Source: CAD feature listing. Evaluate the final solid. Frame: model axes, mm. A direction names the side the tool comes from. Give positions to 0.01 mm unless a question says otherwise; leave off trailing zeros. Loops run counter-clockwise (first coordinate to the right, second up) from the corner with the lowest first, then second, coordinate; pieces in that order, holes last.
from build123d import *

# Parameters (mm, degrees)
BOSS_EXTRUDE1_DEPTH = 50
SKETCH2_W           = 9
SKETCH2_H           = 2
BOSS_EXTRUDE2_DEPTH = 10
SKETCH3_R           = 3.15
CUT_EXTRUDE1_DEPTH  = 1
BOSS_EXTRUDE3_DEPTH = 50
SKETCH5_W           = 5
SKETCH5_H           = 2
BOSS_EXTRUDE4_DEPTH = 1
SKETCH6_R           = 4.5
SKETCH6_R_2         = 2.5
CUT_EXTRUDE2_DEPTH  = 1
CUT_EXTRUDE3_DEPTH  = 65.610577824


with BuildPart() as part:
    # Sketch1 → Boss-Extrude1 (new body)
    with BuildSketch(Plane(origin=(0, 0, 0), x_dir=(1, 0, 0), z_dir=(0, 1, 0))):
        Polygon((0, 0), (0, -6), (7, -6), (7, -4), (2, -4), (2, -2), (9, -2), (9, 0), align=None)
    extrude(amount=BOSS_EXTRUDE1_DEPTH)

    # Sketch2 → Boss-Extrude2 (add)
    with BuildSketch(Plane(origin=(0, 50, 0), x_dir=(1, 0, 0), z_dir=(0, 1, 0))):
        with Locations((4.5, -1)):
            Rectangle(SKETCH2_W, SKETCH2_H)
    extrude(amount=BOSS_EXTRUDE2_DEPTH)

    # Sketch3 → Cut-Extrude1 (cut)
    with BuildSketch(Plane(origin=(0, 0, 0), x_dir=(-1, 0, 0), z_dir=(0, 0, -1))):
        with Locations((-5.5, 55)):
            Circle(SKETCH3_R)
    extrude(amount=-CUT_EXTRUDE1_DEPTH, mode=Mode.SUBTRACT)

    # Sketch4 → Boss-Extrude3 (add)
    with BuildSketch(Plane.XZ):
        Polygon((17.441727636, 16.441727636), (7, 6), (0, 13), (10.857923623, 23.349178451), align=None)
        Polygon((7, 6), (0, 13), (0, 6), align=None)
    extrude(amount=-BOSS_EXTRUDE3_DEPTH)

    # Sketch5 → Boss-Extrude4 (add)
    with BuildSketch(Plane.XZ):
        with Locations((4.5, 3)):
            Rectangle(SKETCH5_W, SKETCH5_H)
    extrude(amount=-BOSS_EXTRUDE4_DEPTH)

    # Sketch6 → Cut-Extrude2 (cut)
    # profile 1 of 2: a face of its own
    with BuildSketch(Plane(origin=(17.350446553, 0, 16.537495917), x_dir=(0.6899452300561162, 0, -0.7238615748351429), z_dir=(0.7238615748351429, 0, 0.6899452300561162))):
        with Locations((-4.638949273, 40)):
            Circle(SKETCH6_R)
        with Locations((-4.638949273, 40)):
            Circle(SKETCH6_R_2, mode=Mode.SUBTRACT)
    # profile 2 of 2: a face of its own
    with BuildSketch(Plane(origin=(17.350446553, 0, 16.537495917), x_dir=(0.6899452300561162, 0, -0.7238615748351429), z_dir=(0.7238615748351429, 0, 0.6899452300561162))):
        with Locations((-4.638949273, 10)):
            Circle(SKETCH6_R)
        with Locations((-4.638949273, 10)):
            Circle(SKETCH6_R_2, mode=Mode.SUBTRACT)
    extrude(amount=-CUT_EXTRUDE2_DEPTH, mode=Mode.SUBTRACT)

    # Sketch6_2 → Cut-Extrude3 (cut, through all)
    with BuildSketch(Plane(origin=(17.350446553, 0, 16.537495917), x_dir=(0.6899452300561162, 0, -0.7238615748351429), z_dir=(0.7238615748351429, 0, 0.6899452300561162))):
        with BuildLine():
            ThreePointArc((-2.138949273, 40), (-2.87118232, 41.767766953), (-4.638949273, 42.5))
            Line((-4.638949273, 42.5), (-4.638949273, 37.5))
            ThreePointArc((-4.638949273, 37.5), (-2.87118232, 38.232233047), (-2.138949273, 40))
        make_face()
        with BuildLine():
            Line((-4.638949273, 37.5), (-4.638949273, 42.5))
            ThreePointArc((-4.638949273, 42.5), (-7.138949273, 40), (-4.638949273, 37.5))
        make_face()
        with BuildLine():
            ThreePointArc((-2.138949273, 10), (-2.87118232, 11.767766953), (-4.638949273, 12.5))
            Line((-4.638949273, 12.5), (-4.638949273, 7.5))
            ThreePointArc((-4.638949273, 7.5), (-2.87118232, 8.232233047), (-2.138949273, 10))
        make_face()
        with BuildLine():
            Line((-4.638949273, 7.5), (-4.638949273, 12.5))
            ThreePointArc((-4.638949273, 12.5), (-7.138949273, 10), (-4.638949273, 7.5))
        make_face()
    extrude(amount=-CUT_EXTRUDE3_DEPTH, mode=Mode.SUBTRACT)


solid = part.part
1) Cut plane B-B (y = 55). Return loops of the section in (x, z), and give its area (3 significant figures).
Checks:
outline: (0, 0) - (2.35, 0) - (2.35, 1) - (8.65, 1) - (8.65, 0) - (9, 0) - (9, 2) - (0, 2) - close
area: 11.7 mm2
2) Cut plane C-C (x = 5.5). State how many separate pieces and enclosed holes the cut face has, and give its area (3 significant figures).
Checks:
separate pieces: 1
enclosed holes: 2
area: 774 mm2
3) Contact query for flat-ended pins moving along their axis: P1, Ø5, axis at x = 13, y = 33.5, coming from the +Z side; P2, Ø2.5, axis at x = 4, y = 25, coming from the +Z side; P3, Ø1.9, axis at x = 4, y = 53.5, coming from the -Z side. Output: stop coordinate, or through.
Checks:
P1: stops at z = 23.35
P2: stops at z = 18
P3: stops at z = 1
4) Ray query, probe 1 along Y at (x, z) = (5.5, 0.65); probe 2 along Z at (x, y) = (8, 9); probe 3 along X at (y, z) = (43, 11.5). Return the intervals inside material, ascending.
Checks:
probe 1: y = 0 to 51.85, 58.15 to 60
probe 2: z = 0 to 2, 7 to 10.87, 17.2 to 20.63
probe 3: x = 0 to 12.5
5) Reachability of faces 4 (the flat face through (12, 25, 11)), 5 (the flat face through (6, 55, 1)), 6 (the flat face through (7, 50, 13)) from +Z, -Z, +X, -X, +Y, -Y: full face, straight path, thin tool, end or side. Return the list, or none.
Checks:
face 4: +X, +Y, -Y
face 5: -Z
face 6: +Z, +X, -X, +Y
6) Pull-direction query (Z, two-part tool) for faces 1 (the flat face through (5.35, 24.65, 18.1)), 2 (the flat face through (5, 30, 2)), 3 (the flat face through (9, 30, 1)); classes: released by +Z, released by -Z, zero draft, split by the parting line, or undercut.
Checks:
face 1: released by +Z
face 2: undercut
face 3: zero draft
7) Cut plane A-A (y = 20.5). Return loops of the section in (x, z), and give its area (3 significant figures).
Checks:
outline: (0, 0) - (9, 0) - (9, 2) - (2, 2) - (2, 4) - (7, 4) - (7, 6) - (17.44, 16.44) - (10.86, 23.35) - (0, 13) - close
area: 205 mm2
